Job drawing, mm, ordinate dimensions from the low corner. One solid piece. Give positions to 0.01 mm unless a question says otherwise; leave off trailing zeros. Loops run counter-clockwise (first coordinate to the right, second up) from the corner with the lowest first, then second, coordinate; pieces in that order, holes last. Notation, with made-up numbers: M 75.5,54.5 L 127.5,54.5 A15 cw 127.5,80.5 Z; hole C 28,-35 d10. An arc over 180 degrees is marked long. Answer as CSV lines item,"result".
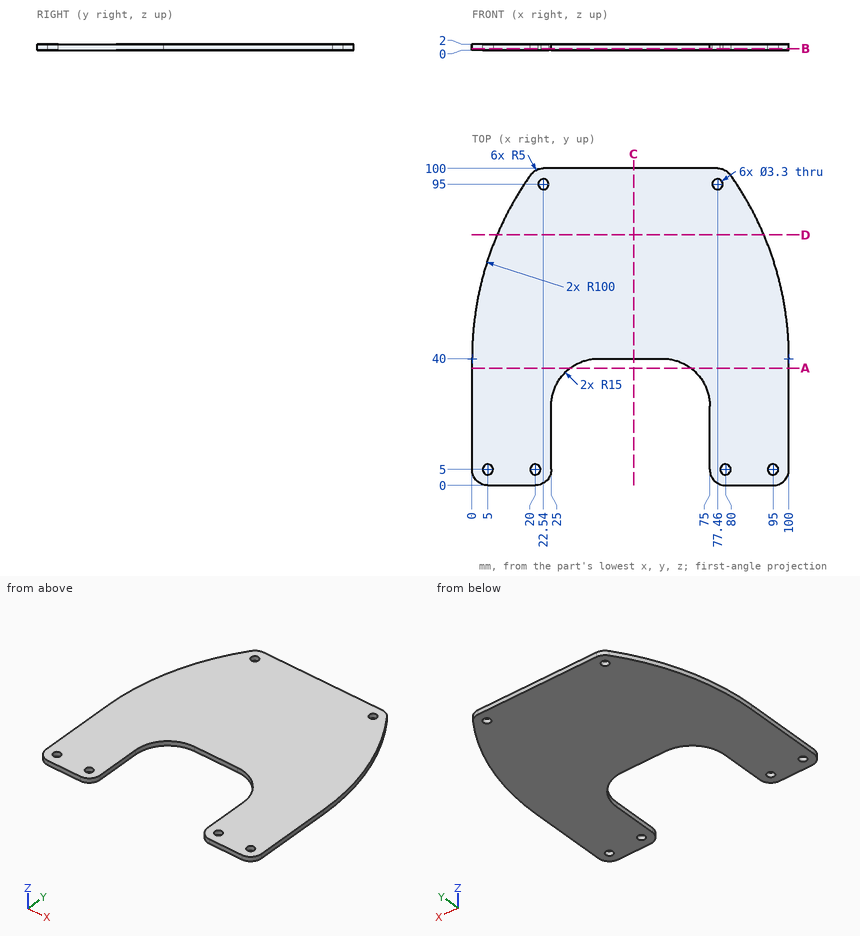
1) Drill centre lines: line 1 (X direction, y = 16, z = 1.95); line 2 (X direction, y = 95, z = 1) (1 decimal); line 3 (Y direction, x = 53, z = 0.3). Where is each one in solid material? Low to high. Write a range as from..to.
Answer below:
line 1,"x = 0..25, 75..100"
line 2,"x = 16.5..20.9, 24.2..75.8, 79.1..83.5"
line 3,"y = 40..100"
2) Band-saw the part on B-B on z = 0.55. Give the number of separate pieces and of enclosed holes in the cut face, and give its area (3 significant figures).
Answer below:
separate pieces,"1"
enclosed holes,"6"
area,"7,260 mm^2"
3) Band-saw the part on A-A on y = 37. Give the cut face in (x, z), and give its area (3 significant figures).
Answer below:
outline,"M 0,0 L 31,0 L 31,2 L 0,2 Z; M 69,0 L 100,0 L 100,2 L 69,2 Z"
area,"124 mm^2"
4) Flat gauge pin, fed straight in: pin 1 (2 mm diameter, centred on x = 77.46, y = 95, fed in from +Z). Where does the tip first touch, or does it go through?
Answer below:
pin 1,"passes through"
5) Band-saw the part on C-C on x = 51. Give the cut face in (y, z).
Answer below:
outline,"M 40,0 L 100,0 L 100,2 L 40,2 Z"
6) Band-saw the part on D-D on y = 79. Give the cut face in (x, z).
Answer below:
outline,"M 7.92,0 L 92.08,0 L 92.08,2 L 7.92,2 Z"
